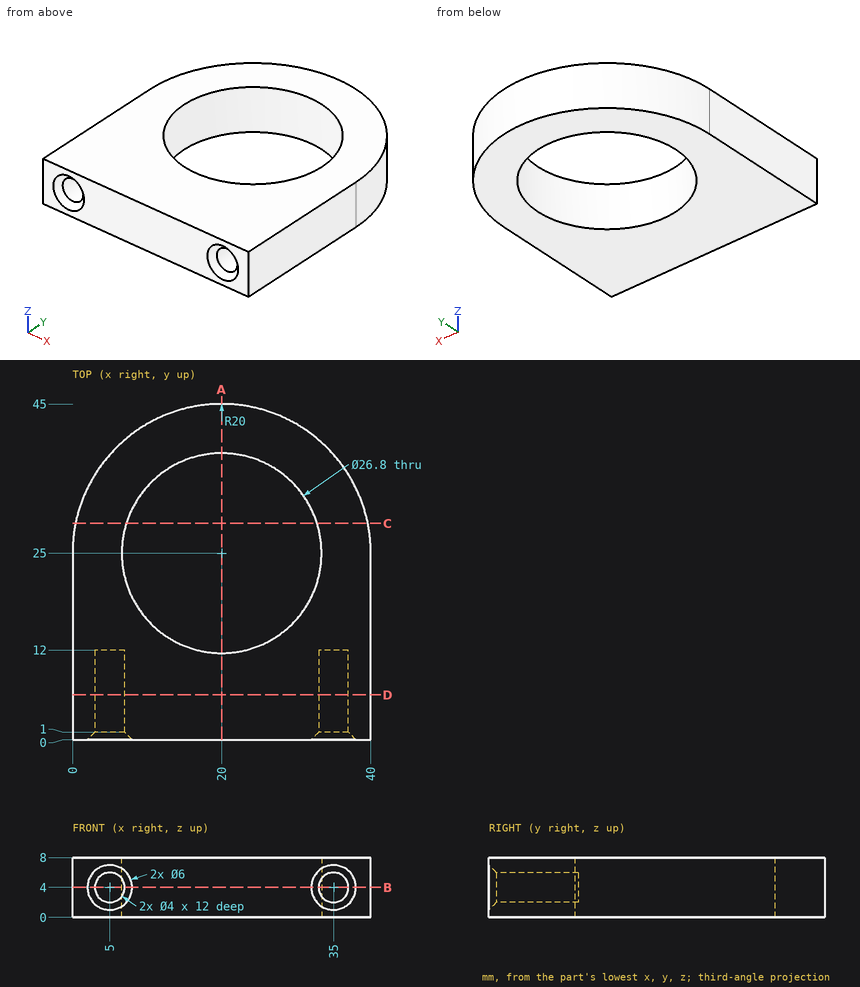
Check sheet for the drawn part. Datum: minimum x, y, z corner. Units: mm. Give positions to 0.01 mm unless a question says otherwise; leave off trailing zeros. Loops run counter-clockwise (first coordinate to the right, second up) from the corner with the lowest first, then second, coordinate; pieces in that order, holes last. Notation, with made-up numbers: M 55.25,-3 L 61.25,-3 A29 ccw 61.25,31 Z; hole C -2,-12 d4. An arc over 180 degrees is marked long. Return JSON: item names as keys, results as strings.
1) Section check B-B, the plane z = 4. Enter the section's corners in (x, y), and give its area (3 significant figures).
Findings:
{"outline": "M 0,0 L 2,0 L 3,1 L 3,12 L 7,12 L 7,1 L 8,0 L 32,0 L 33,1 L 33,12 L 37,12 L 37,1 L 38,0 L 40,0 L 40,25 A20 ccw 0,25 Z; hole C 20,25 d26.8", "area": "966 mm2"}
2) Section check D-D, the plane y = 6. Enter the section's corners in (x, z), and give its area (3 significant figures).
Findings:
{"outline": "M 0,0 L 40,0 L 40,8 L 0,8 Z; hole C 5,4 d4; hole C 35,4 d4", "area": "295 mm2"}
3) Section check A-A, the plane x = 20. Enter the section's corners in (y, z).
Findings:
{"outline": "M 0,0 L 11.6,0 L 11.6,8 L 0,8 Z; M 38.4,0 L 45,0 L 45,8 L 38.4,8 Z"}
4) Material ranges on L1, parallel to Z at x = 5, y = 7.5; L2, parallel to Y at x = 20, z = 2.75; L3, parallel to Y at x = 32, z = 7.5, recorded low to high. Write a range as [from, to].
Findings:
{"L1": "z = [0, 2], [6, 8]", "L2": "y = [0, 11.6], [38.4, 45]", "L3": "y = [0, 19.04], [30.96, 41]"}
5) Section check C-C, the plane y = 29. Enter the section's corners in (x, z).
Findings:
{"outline": "M 0.4,0 L 7.21,0 L 7.21,8 L 0.4,8 Z; M 32.79,0 L 39.6,0 L 39.6,8 L 32.79,8 Z"}
6) Gauge pin test, flat ends, axial feed: P1, Ø1.2, axis at x = 4.5, z = 4, coming from the -Y side; P2, Ø1.5, axis at x = 31.5, z = 4.5, coming from the -Y side; P3, Ø2, axis at x = 34, z = 3.5, coming from the -Y side; P4, Ø4.5, axis at x = 35, z = 4, coming from the -Y side. Record the tip position at first contact, or that the pin passes through.
Findings:
{"P1": "stops at y = 12", "P2": "stops at y = 0", "P3": "stops at y = 0.88", "P4": "stops at y = 0.75"}
